```python
from build123d import *

# Parameters (mm, degrees)
SKETCH_1_W               = 14
SKETCH_1_H               = 5.2
EXTRUDE_1_DEPTH          = 50
SKETCH_3_R               = 2.75
CUT_EXTRUDE_1_DEPTH      = 3
CUT_EXTRUDE_2_DEPTH      = 51.754704215
CUT_EXTRUDE_2_DEPTH_BACK = 51.754704215
SKETCH_4_R               = 1.5


with BuildPart() as part:
    # 草图1 → 凸台-拉伸1 (new, symmetric)
    with BuildSketch(Plane.XY):
        Rectangle(SKETCH_1_W, SKETCH_1_H)
    extrude(amount=EXTRUDE_1_DEPTH, both=True)

    # 草图3 → 切除-拉伸1 (cut)
    with BuildSketch(Plane(origin=(0, 2.6, 0), x_dir=(1, 0, 0), z_dir=(0, 1, 0))):
        with Locations(Location((0, -45, 0), (0, 0, 270))):
            Circle(SKETCH_3_R)
        with Locations(Location((0, -15, 0), (0, 0, 270))):
            Circle(SKETCH_3_R)
        with Locations(Location((0, 15, 0), (0, 0, 270))):
            Circle(SKETCH_3_R)
        with Locations(Location((0, 45, 0), (0, 0, 270))):
            Circle(SKETCH_3_R)
    extrude(amount=-CUT_EXTRUDE_1_DEPTH, mode=Mode.SUBTRACT)

    # 草图4 → 切除-拉伸2 (cut, two sides: drawn at the far end of the back side and taken through both)
    with BuildSketch(Plane(origin=(0, 2.6, 0), x_dir=(1, 0, 0), z_dir=(0, 1, 0)).offset(-CUT_EXTRUDE_2_DEPTH_BACK)):
        with Locations(Location((0, -45, 0), (0, 0, 270))):
            Circle(SKETCH_4_R)
        with Locations(Location((0, -15, 0), (0, 0, 270))):
            Circle(SKETCH_4_R)
        with Locations(Location((0, 15, 0), (0, 0, 270))):
            Circle(SKETCH_4_R)
        with Locations(Location((0, 45, 0), (0, 0, 270))):
            Circle(SKETCH_4_R)
    extrude(amount=CUT_EXTRUDE_2_DEPTH + CUT_EXTRUDE_2_DEPTH_BACK, mode=Mode.SUBTRACT)


solid = part.part
```
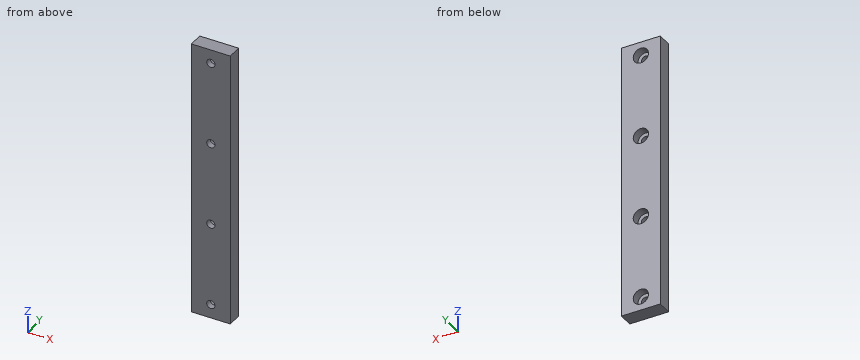
Read the model definition and answer for the solid it produces. Units are mm, in the model's axes. Give positions to 0.01 mm unless a question says otherwise; leave off trailing zeros. Write each loop counter-clockwise with the first axis right and the second up, starting at its lowest first coordinate (ties: lowest second). Pieces come first, ordered by that corner, then holes. Notation, with made-up numbers: (57, 2) - (99, 2) arc R35 ccw to (99, 40) - close; hole circle Ø4 at (15, 27). An arc over 180 degrees is marked (long way). Write item = value, one per line. Start each with the question number.
Item 1: Find the intervals of material crossed by probe 1 along Z at (x, y) = (0, -1.7); probe 2 along X at (y, z) = (-1.5, 45); probe 3 along X at (y, z) = (0.65, 15), in increasing order. Write a range as [from, to].
Item 2: Find section A-A (y = 1). Give the vertices of the cut face in (x, z), then the cut area to 3 significant figures.
Item 3: Find section B-B (z = -45). Give the vertices of the cut face in (x, y), then the cut area to 3 significant figures.
Item 4: Find section C-C (x = 0). State how many separate pieces and enclosed holes the cut face has, then the cut area to 3 significant figures.
Item 5: Each of these flat-tipped pins is pushed along its axis until it touches: P1, Ø4.5, axis at x = 0, z = 15, coming from the +Y side; P2, Ø5, axis at x = 0, z = 45, coming from the -Y side. Where does it stop, or does it pass through?
Response:
q1.probe_1 = [-50, -46.5], [-43.5, -16.5], [-13.5, 13.5], [16.5, 43.5], [46.5, 50]
q1.probe_2 = [-7, -1.5], [1.5, 7]
q1.probe_3 = [-7, -2.75], [2.75, 7]
q2.outline = (-7, -50) - (7, -50) - (7, 50) - (-7, 50) - close; hole circle Ø5.5 at (0, -45); hole circle Ø5.5 at (0, -15); hole circle Ø5.5 at (0, 15); hole circle Ø5.5 at (0, 45)
q2.area = 1,300 mm²
q3.outline = (-7, -2.6) - (-1.5, -2.6) - (-1.5, -0.4) - (-2.75, -0.4) - (-2.75, 2.6) - (-7, 2.6) - close; (1.5, -2.6) - (7, -2.6) - (7, 2.6) - (2.75, 2.6) - (2.75, -0.4) - (1.5, -0.4) - close
q3.area = 49.7 mm²
q4.separate_pieces = 5
q4.enclosed_holes = 0
q4.area = 428 mm²
q5.P1 = -0.4
q5.P2 = -2.6
